Check sheet for the modelled part. Datum: model origin and axes. Units: mm. Face numbers are marked on the shaded views. Give positions to 0.01 mm unless a question says otherwise; leave off trailing zeros. Order: outer loops, then holes, each group sorted by start corner. A loop starts at its lowest first (then second) coordinate and runs counter-clockwise, first axis right, second up.
from build123d import *

# Parameters (mm, degrees)
F0_R          = 39.6875
F0_R_2        = 38.1
F1_DEPTH      = 30
F2_W          = 25.0000006067
F2_H          = 20
F3_DEPTH      = 37.846
F3_DEPTH_BACK = 26.416
F4_W          = 36.5361310542
F4_H          = 63.4360015392
F5_DEPTH      = 7.5
F6_R          = 1.7228830897
F6_R_2        = 2.0395757716
F7_DEPTH      = 25.4
F7_DEPTH_BACK = 13.462
F8_R          = 1.7580369287
F8_R_2        = 1.6852602443
F9_DEPTH      = 50


with BuildPart() as f1:
    # F0 (on Top) → F1 (new body)
    with BuildSketch(Plane.XY):
        Circle(F0_R)
        Circle(F0_R_2, mode=Mode.SUBTRACT)
    extrude(amount=F1_DEPTH)

    # F2 (on Right) → F3 (cut, two sides)
    with BuildSketch(Plane.YZ) as f3_sk:
        with Locations((34.4710433856, 14.9242004845)):
            Rectangle(F2_W, F2_H)
    extrude(amount=-F3_DEPTH, mode=Mode.SUBTRACT)
    extrude(f3_sk.sketch, amount=F3_DEPTH_BACK, mode=Mode.SUBTRACT)

    # F4 (on Right) → F5 (cut)
    with BuildSketch(Plane.YZ):
        with Locations((49.4740214199, 27.9371961951)):
            Rectangle(F4_W, F4_H)
    extrude(amount=-F5_DEPTH, mode=Mode.SUBTRACT)

    # F6 (on Front) → F7 (cut, two sides)
    with BuildSketch(Plane.XZ) as f7_sk:
        with Locations((-17.5434835255, -25.1583587378)):
            Circle(F6_R)
        with Locations((-17.5434835255, 0)):
            Circle(F6_R_2)
    extrude(amount=-F7_DEPTH, mode=Mode.SUBTRACT)
    extrude(f7_sk.sketch, amount=F7_DEPTH_BACK, mode=Mode.SUBTRACT)

    # F8 (on Front) → F9 (cut)
    with BuildSketch(Plane.XZ):
        with Locations((2.758965129, 27.4874716997)):
            Circle(F8_R)
        with Locations((2.758965129, 2.3502300028)):
            Circle(F8_R_2)
    extrude(amount=-F9_DEPTH, mode=Mode.SUBTRACT)


solid = f1.part
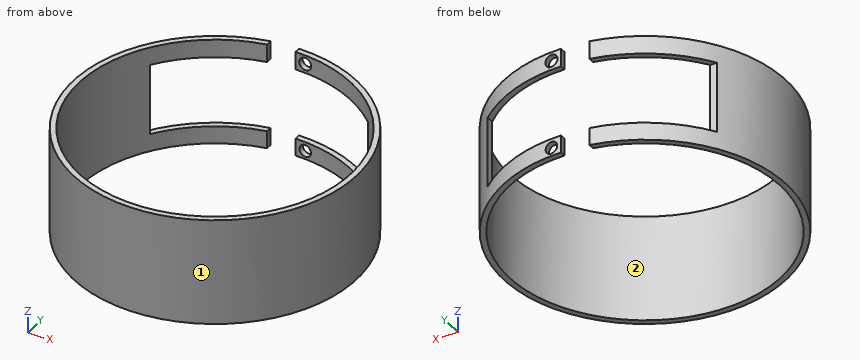
1) Draft check along Y on the marked faces 1 and 2. Enter one of: +Y half, -Y half, draft (parallel to the pull), parting line (faces both ways), or undercut.
Recorded:
face 1: parting line
face 2: undercut
2) Section check A-A, the plane y = -29. Record the cut outline in (x, z), then the cut area to 3 significant figures.
Recorded:
outline: (-27.09, 0) - (-24.71, 0) - (-24.71, 30) - (-27.09, 30) - close; (24.71, 0) - (27.09, 0) - (27.09, 30) - (24.71, 30) - close
area: 143 mm2
3) Section check D-D, the plane x = 2.5. Record the cut outline in (y, z).
Recorded:
outline: (-39.61, 0) - (-38.02, 0) - (-38.02, 30) - (-39.61, 30) - close; (38.02, 0) - (39.61, 0) - (39.61, 0.68) - (38.02, 0.68) - close; (38.02, 4.02) - (39.61, 4.02) - (39.61, 4.92) - (38.02, 4.92) - close; (38.02, 24.92) - (39.61, 24.92) - (39.61, 25.75) - (38.02, 25.75) - close; (38.02, 29.23) - (39.61, 29.23) - (39.61, 30) - (38.02, 30) - close
4) Section check C-C, the plane x = 33. Record the cut outline in (y, z), then the cut area to 3 significant figures.
Recorded:
outline: (-22.05, 0) - (-19.04, 0) - (-19.04, 30) - (-22.05, 30) - close; (19.04, 0) - (22.05, 0) - (22.05, 30) - (19.04, 30) - close
area: 180 mm2
5) Depth check by flat-ended pin: pin 1 Ø0.6 at (x, z) = (-31.5, 10.5) entering from +Y; pin 2 Ø5 at (y, z) = (-23.5, 20) entering from -X; pin 3 Ø5 at (x, z) = (-27.5, 14) entering from +Y; pin 4 Ø2 at (x, z) = (1, 19) entering from -Y. Enter the tip coordinate at first touch or a pass-through.
Recorded:
pin 1: stops at y = 21.97
pin 2: stops at x = -33.68
pin 3: stops at y = -23.49
pin 4: stops at y = -39.69
6) Material ranges on L1, parallel to X at y = 0, z = 10; L2, parallel to X at y = 29, z = 27.5; L3, parallel to X at y = 24, z = 5, recorded low to high.
Recorded:
L1: x = -39.69 to -38.1, 38.1 to 39.69
L2: x = -27.09 to -24.71, 24.71 to 27.09
L3: x = 29.59 to 31.61
7) Section check B-B, the plane x = -25. Record the cut outline in (y, z), then the cut area to 3 significant figures.
Recorded:
outline: (-30.82, 0) - (-28.75, 0) - (-28.75, 30) - (-30.82, 30) - close; (28.75, 0) - (30.82, 0) - (30.82, 4.92) - (28.75, 4.92) - close; (28.75, 24.92) - (30.82, 24.92) - (30.82, 30) - (28.75, 30) - close
area: 82.9 mm2
